Autodesk Inventor part; units mm, degrees
ref_plane "YZ Plane" through (0, 0, 0) normal (1, 0, 0) x (0, 1, 0)
ref_plane "XZ Plane" through (0, 0, 0) normal (0, 1, 0) x (-1, 0, 0)
ref_plane "XY Plane" through (0, 0, 0) normal (0, 0, 1) x (1, 0, 0)
sketch "Sketch1" plane through (0, 0, 0) normal (1, 0, 0) x (0, 1, 0)
  line L0 (-31.5, 40) -> (31.5, 40)
  line L1 (31.5, 40) -> (31.5, -40)
  line L2 (31.5, -40) -> (-31.5, -40)
  line L3 (-31.5, -40) -> (-31.5, 40)
  line L4 (-31.5, 40) -> (31.5, -40) construction
  line L5 (31.5, 40) -> (-31.5, -40) construction
  point P0 (0, 0)
  dimension "d0" = 63
  dimension "d1" = 80
extrude "Extrusion1" add sketch "Sketch1" along normal blind 3
sketch "Sketch2" plane through (3, 0, 0) normal (1, 0, 0) x (0, 0, -1)
  line L0 (40, -31.5) -> (40, 31.5)
  line L1 (40, 31.5) -> (37, 31.5)
  line L2 (37, 31.5) -> (37, -1.5)
  line L3 (37, -1.5) -> (40, -1.5)
  line L4 (40, -1.5) -> (40, 31.5)
  line L5 (-40, -31.5) -> (40, -31.5)
  line L6 (0, -31.5) -> (20, -31.5)
  line L7 (20, -31.5) -> (20, -28.5)
  line L8 (20, -28.5) -> (0, -28.5)
  line L9 (0, -28.5) -> (0, -31.5)
  line L10 (-37, -31.5) -> (-20, -31.5)
  line L11 (-20, -31.5) -> (-20, -28.5)
  line L12 (-20, -28.5) -> (-37, -28.5)
  line L13 (-37, -28.5) -> (-37, -31.5)
  point P0 (0, 0)
  dimension "d4" = 3
  dimension "d5" = 30
  dimension "d6" = 20
  dimension "d7" = 3
  dimension "d8" = 20
  dimension "d9" = 17
  dimension "d10" = 3
  dimension "d11" = 20
extrude "Extrusion2" cut sketch "Sketch2" against normal through all
sketch "Sketch3" plane through (3, 0, 0) normal (1, 0, 0) x (0, 0, -1)
  line L0 (-40, 31.5) -> (-40, -31.5)
  line L1 (-40, 31.5) -> (-37, 31.5)
  line L2 (-37, 31.5) -> (-37, -1.5)
  line L3 (-37, -1.5) -> (-40, -1.5)
  line L4 (-40, -1.5) -> (-40, 31.5)
  point P0 (0, 0)
  dimension "d14" = 3
  dimension "d15" = 33
extrude "Extrusion3" cut sketch "Sketch3" against normal through all
sketch "Sketch4" plane through (3, 0, 0) normal (1, 0, 0) x (0, 0, -1)
  line L0 (37, 31.5) -> (-37, 31.5)
  line L1 (0, 31.5) -> (20, 31.5)
  line L2 (20, 31.5) -> (20, 28.5)
  line L3 (20, 28.5) -> (0, 28.5)
  line L4 (0, 28.5) -> (0, 31.5)
  line L5 (37, -1.5) -> (37, 31.5)
  point P0 (0, 0)
  dimension "d18" = 20
  dimension "d19" = 3
  dimension "d20" = 17
extrude "Extrusion4" cut sketch "Sketch4" against normal through all
properties part number "side"
Input: part model. Units: mm. Frame: model coordinates. A direction names the side the tool comes from. Coordinates: 2 decimals unless noted, no trailing zeros. Write each loop counter-clockwise with the first axis right and the second up, starting at its lowest first coordinate (ties: lowest second). Pieces come first, ordered by that corner, then holes. Notation, with made-up numbers: (10.5, 73) -> (58.5, 73) arc R32 ccw to (58.5, 104) -> close; hole circle Ø2 at (43.25, 16.25). An arc over 180 degrees is marked (long way). Answer as a JSON object with one key per item and string values.
1. Mould query, pull axis Z, two halves, no side actions, for faces 1 (the face through (2, -1.5, -38)), 2 (the face through (2, -30, 37)), 3 (the face through (2, 15, -37)). Classes: released by +Z, released by -Z, zero draft, split by the parting line, or undercut.
Result set:
{"face 1": "zero draft", "face 2": "undercut", "face 3": "released by -Z"}
2. Access query for faces 4 (the face through (2, 30, -20)), 5 (the face through (2, -1.5, 38)), 6 (the face through (2, -30, 0)). Directions: +Z, -Z, +X, -X, +Y, -Y. A direction counts if a zero-diameter tool reaches every point of the face in a straight line with its end or side. Return the directions, or none.
Result set:
{"face 4": "+X, -X, +Y", "face 5": "+Z, +X, -X, +Y", "face 6": "+X, -X, -Y"}
3. First-contact query: P1, Ø1.5, axis at x = 1, z = -38.5, coming from the +Y side; P2, Ø0.9, axis at x = 1, z = 28, coming from the -Y side; P3, Ø1.5, axis at x = 1.5, y = 18.5, coming from the +Z side; P4, Ø5, axis at y = 1.5, z = -1.5, coming from the -X side. Flat tips, straight axial feed; report the tip coordinate or a pass-through.
Result set:
{"P1": "stops at y = -1.5", "P2": "stops at y = -28.5", "P3": "stops at z = 37", "P4": "stops at x = 0"}
4. Section C-C on y = 2. Return the cut outline in (x, z), then the cut area to 3 significant figures.
Result set:
{"outline": "(0, -37) -> (3, -37) -> (3, 37) -> (0, 37) -> close", "area": "222 mm2"}
5. Section A-A on x = 1.6. Return the cut outline in (y, z).
Result set:
{"outline": "(-31.5, -40) -> (-1.5, -40) -> (-1.5, -37) -> (31.5, -37) -> (31.5, -20) -> (28.5, -20) -> (28.5, 0) -> (31.5, 0) -> (31.5, 37) -> (-1.5, 37) -> (-1.5, 40) -> (-31.5, 40) -> (-31.5, 37) -> (-28.5, 37) -> (-28.5, 20) -> (-31.5, 20) -> (-31.5, 0) -> (-28.5, 0) -> (-28.5, -20) -> (-31.5, -20) -> close"}
6. Section B-B on z = 32.5. Return the cut outline in (x, y), then the cut area to 3 significant figures.
Result set:
{"outline": "(0, -28.5) -> (3, -28.5) -> (3, 31.5) -> (0, 31.5) -> close", "area": "180 mm2"}
7. Material intervals for line 1 (Z direction, x = 1.35, y = 29.5); line 2 (Z direction, x = 0.85, y = 4.5); line 3 (Y direction, x = 2, z = -15.5), sorted ascending. Write a range as from..to.
Result set:
{"line 1": "z = -37..-20, 0..37", "line 2": "z = -37..37", "line 3": "y = -28.5..28.5"}
